Input: part model. Units: mm. Frame: model coordinates. Face numbers are marked on the shaded views. Give positions to 0.01 mm unless a question says otherwise; leave off trailing zeros. Order: outer loops, then holes, each group sorted by start corner. A loop starts at its lowest first (then second) coordinate and runs counter-clockwise, first axis right, second up. Notation, with made-up numbers: (63, 77.25) - (99, 77.25) arc R36 cw to (99, 116.25) - close; hole circle Ø4 at (14, -13.75). An arc over 180 degrees is marked (long way). Use a Markdown table: item, result.
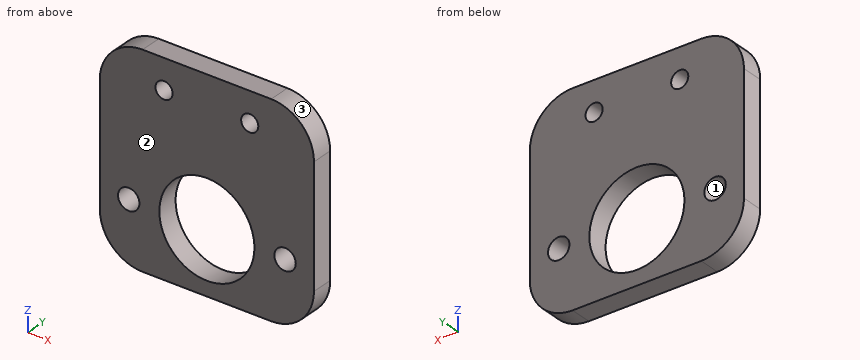
from build123d import *

# Parameters (mm, degrees)
ESBO_O1_W                = 50
ESBO_O1_H                = 48
RESSALTO_EXTRUS_O1_DEPTH = 5
ESBO_O2_R                = 11.1
ESBO_O2_R_2              = 2.5
CORTE_EXTRUS_O1_DEPTH    = 5
FILETE1_R                = 10
FILETE2_R                = 10
FILETE3_R                = 10
FILETE4_R                = 10
ESBO_O3_R                = 2
CORTE_EXTRUS_O2_DEPTH    = 22


with BuildPart() as part:
    # Esboço1 → Ressalto-extrusão1 (new body)
    with BuildSketch(Plane(origin=(0, 0, 0), x_dir=(1, 0, 0), z_dir=(0, 1, 0))):
        with Locations((25, 24)):
            Rectangle(ESBO_O1_W, ESBO_O1_H)
    extrude(amount=RESSALTO_EXTRUS_O1_DEPTH)

    # Esboço2 → Corte-extrusão1 (cut)
    with BuildSketch(Plane(origin=(0, 5, 0), x_dir=(1, 0, 0), z_dir=(0, 1, 0))):
        with Locations(Location((25, 33.5, 0), (0, 0, 270))):
            Circle(ESBO_O2_R)
        with Locations(Location((6.75, 33.5, 0), (0, 0, 270))):
            Circle(ESBO_O2_R_2)
        with Locations(Location((43.25, 33.5, 0), (0, 0, 90))):
            Circle(ESBO_O2_R_2)
    extrude(amount=-CORTE_EXTRUS_O1_DEPTH, mode=Mode.SUBTRACT)

    # Filete1
    filete1_edges = [part.edges().sort_by_distance(p)[0] for p in [
        (50, 2.5, 0),
    ]]
    fillet(filete1_edges, radius=FILETE1_R)

    # Filete2
    filete2_edges = [part.edges().sort_by_distance(p)[0] for p in [
        (0, 2.5, 0),
    ]]
    fillet(filete2_edges, radius=FILETE2_R)

    # Filete3
    filete3_edges = [part.edges().sort_by_distance(p)[0] for p in [
        (50, 2.5, -48),
    ]]
    fillet(filete3_edges, radius=FILETE3_R)

    # Filete4
    filete4_edges = [part.edges().sort_by_distance(p)[0] for p in [
        (0, 2.5, -48),
    ]]
    fillet(filete4_edges, radius=FILETE4_R)

    # Esboço3 → Corte-extrusão2 (cut)
    with BuildSketch(Plane(origin=(0, 5, 0), x_dir=(1, 0, 0), z_dir=(0, 1, 0))):
        with Locations(Location((15, 7, 0), (0, 0, 270))):
            Circle(ESBO_O3_R)
        with Locations(Location((35, 7, 0), (0, 0, 90))):
            Circle(ESBO_O3_R)
    extrude(amount=-CORTE_EXTRUS_O2_DEPTH, mode=Mode.SUBTRACT)


solid = part.part
1. Material intervals for line 1 along X through (y, z) = (1.9, -33.5); line 2 along Z through (x, y) = (35, 3.8); line 3 along X through (y, z) = (2.5, -32), sorted ascending.
Response:
| item | result |
|---|---|
| line 1 | x = 0 to 4.25, 9.25 to 13.9, 36.1 to 40.75, 45.75 to 50 |
| line 2 | z = -48 to -38.32, -28.68 to -9, -5 to 0 |
| line 3 | x = 0 to 4.75, 8.75 to 14, 36 to 41.25, 45.25 to 50 |
2. Section query D-D (z = -23). Return loops of the section in (x, y), then the cut area to 3 significant figures.
Response:
| item | result |
|---|---|
| outline | (0, 0) - (21.4, 0) - (21.4, 5) - (0, 5) - close; (28.6, 0) - (50, 0) - (50, 5) - (28.6, 5) - close |
| area | 214 mm^2 |
3. Section query B-B (x = 25). Return loops of the section in (y, z).
Response:
| item | result |
|---|---|
| outline | (0, -48) - (5, -48) - (5, -44.6) - (0, -44.6) - close; (0, -22.4) - (5, -22.4) - (5, 0) - (0, 0) - close |
4. Mould query, pull axis Z, two halves, no side actions, for the marked faces 1, 2 and 3. Classes: pulls with the +Z half, pulls with the -Z half, needs draft (parallel to the pull), parting line crosses it, or undercut.
Response:
| item | result |
|---|---|
| face 1 | undercut |
| face 2 | needs draft |
| face 3 | pulls with the +Z half |
5. Pin query (flat end, axial travel): pin 1 (8 mm diameter, centred on x = 21.5, z = -32, fed in from -Y). Return the tip coordinate at first contact, or that it passes through.
Response:
| item | result |
|---|---|
| pin 1 | passes through |
6. Section query C-C (y = 2.5). Return loops of the section in (x, z), then the cut area to 3 significant figures.
Response:
| item | result |
|---|---|
| outline | (0, -38) arc R10 ccw to (10, -48) - (40, -48) arc R10 ccw to (50, -38) - (50, -10) arc R10 ccw to (40, 0) - (10, 0) arc R10 ccw to (0, -10) - close; hole circle Ø5 at (6.75, -33.5); hole circle Ø4 at (15, -7); hole circle Ø22.2 at (25, -33.5); hole circle Ø4 at (35, -7); hole circle Ø5 at (43.25, -33.5) |
| area | 1,860 mm^2 |
7. Section query A-A (z = -33.5). Return loops of the section in (x, y), then the cut area to 3 significant figures.
Response:
| item | result |
|---|---|
| outline | (0, 0) - (4.25, 0) - (4.25, 5) - (0, 5) - close; (9.25, 0) - (13.9, 0) - (13.9, 5) - (9.25, 5) - close; (36.1, 0) - (40.75, 0) - (40.75, 5) - (36.1, 5) - close; (45.75, 0) - (50, 0) - (50, 5) - (45.75, 5) - close |
| area | 89.0 mm^2 |
